The drawing under review shows one solid part. Ordinate dimensions are in mm from its lowest x, y, z. A direction names the side the tool comes from. Coordinates: 2 decimals unless noted, no trailing zeros. Write each loop counter-clockwise with the first axis right and the second up, starting at its lowest first coordinate (ties: lowest second). Pieces come first, ordered by that corner, then holes.
1) We need section A-A on x = 3. Write out the cut boundary in (y, z), then the cut area to 3 significant figures.
2) We need section C-C on z = 6.25. Write out the cut boundary in (x, y), then the cut area to 3 significant figures.
3) For the marked faces 1 and 2, list the 3-axis set-ups (+Z, -Z, +X, -X, +Y, -Y) from which the entire face can be reached by the end or side of a thin tool; tool diameter is ignored.
4) Insertion check: P1, Ø1, axis at x = 3, z = 4.5, coming from the -Y side; P2, Ø1.5, axis at y = 4.5, z = 5.5, coming from the -X side; P3, Ø2, axis at y = 1, z = 6.5, coming from the +X side. Each pin has a flat end and moves straight along its axis. Give the tip position at first contact, or say it passes through.
5) To check wall thickness, follow line 1 along Z through (x, y) = (3.85, 1); line 2 along Y through (x, z) = (1.7, 8); line 3 along Y through (x, z) = (2.6, 2.25). State the ranges of each line that lie inside material, in increasing order.
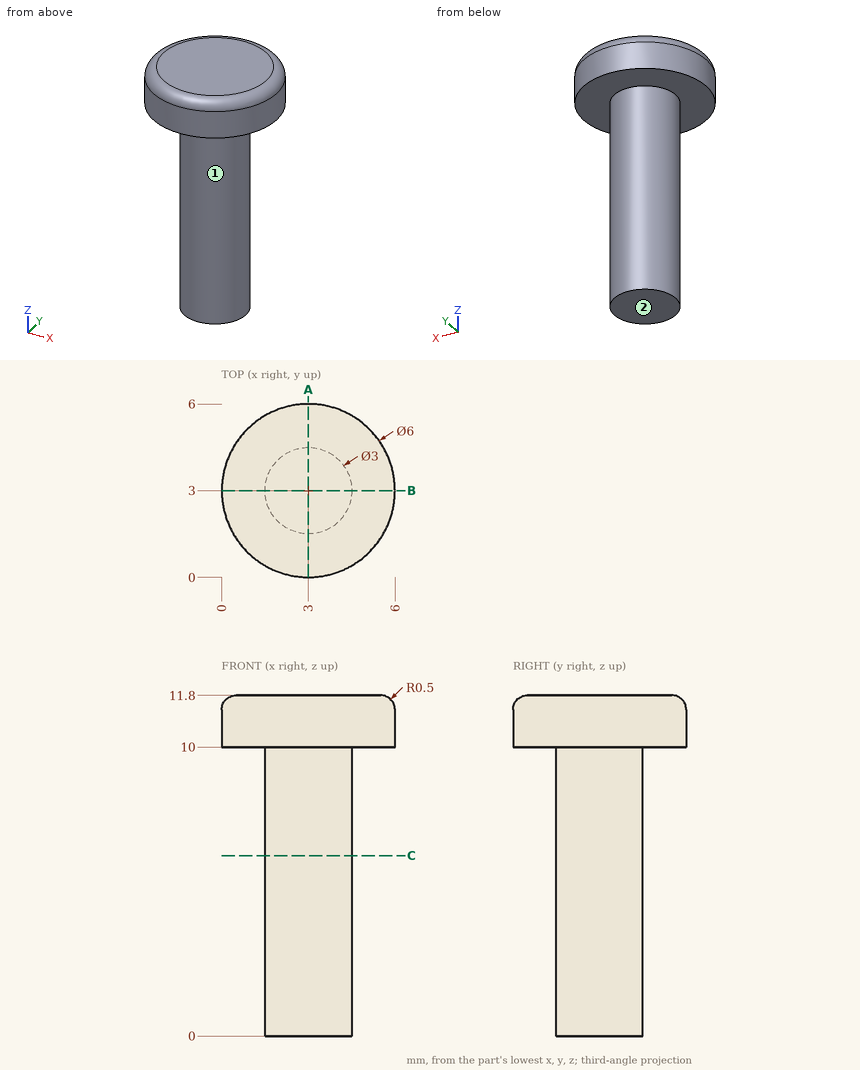
Result:
1. outline: (0, 10) - (1.5, 10) - (1.5, 0) - (4.5, 0) - (4.5, 10) - (6, 10) - (6, 11.3) arc R0.5 ccw to (5.5, 11.8) - (0.5, 11.8) arc R0.5 ccw to (0, 11.3) - close
1. area: 40.7 mm2
2. outline: circle Ø3 at (3, 3)
2. area: 7.07 mm2
3. face 1: -Z
3. face 2: -Z, +X, -X, +Y, -Y
4. P1: stops at y = 1.5
4. P2: stops at x = 1.7
4. P3: stops at x = 4.12
5. line 1: z = 10 to 11.8
5. line 2: y = 2.25 to 3.75
5. line 3: y = 1.55 to 4.45
